from build123d import *

# Parameters (mm, degrees)
BOSS_EXTRUDE1_DEPTH                                  = 5
SKETCH2_W                                            = 20
SKETCH2_H                                            = 6
BOSS_EXTRUDE2_DEPTH                                  = 30
SKETCH3_R                                            = 1.5
CUT_EXTRUDE1_DEPTH                                   = 50.558046773
REFRENTADO_PARA_TORNILLO_CON_CABEZA_PLAN_D           = 3.4
REFRENTADO_PARA_TORNILLO_CON_CABEZA_PLAN_CBORE_D     = 6.5
REFRENTADO_PARA_TORNILLO_CON_CABEZA_PLAN_CBORE_DEPTH = 2
CUT_EXTRUDE2_REACH                                   = 47
SKETCH7_R                                            = 2.5
TALADRO_DE_MARGEN_PARA_M51_D                         = 5.3
TALADRO_DE_MARGEN_PARA_M51_DEPTH                     = 5
TALADRO_DE_MARGEN_PARA_M51_TIP                       = 1.59228064


with BuildPart() as part:
    # Sketch1 → Boss-Extrude1 (new body)
    with BuildSketch(Plane(origin=(0, 0, 0), x_dir=(1, 0, 0), z_dir=(0, 1, 0))):
        Polygon((0, 0), (-20, 0), (-20, -20), (0, -20), (20, -20), (20, 0), (20, 20), (0, 20), align=None)
    extrude(amount=-BOSS_EXTRUDE1_DEPTH)

    # Sketch2 → Boss-Extrude2 (add)
    with BuildSketch(Plane(origin=(0, 0, 0), x_dir=(1, 0, 0), z_dir=(0, 1, 0))):
        with Locations((10, 17)):
            Rectangle(SKETCH2_W, SKETCH2_H)
    extrude(amount=BOSS_EXTRUDE2_DEPTH)

    # Sketch3 → Cut-Extrude1 (cut, through all)
    with BuildSketch(Plane.XY.offset(-14)):
        with Locations((2.5, 7)):
            Circle(SKETCH3_R)
        with Locations(Location((2.5, 23, 0), (0, 0, 180))):
            Circle(SKETCH3_R)
        with Locations(Location((17.5, 7, 0), (0, 0, 180))):
            Circle(SKETCH3_R)
        with Locations((17.5, 23)):
            Circle(SKETCH3_R)
    extrude(amount=-CUT_EXTRUDE1_DEPTH, mode=Mode.SUBTRACT)

    # Refrentado para tornillo con cabeza plana de M31 (through all)
    with Locations(Plane.XY.offset(-14)):
        with Locations((2.5, 23), (2.5, 7), (17.5, 7), (17.5, 23)):
            CounterBoreHole(REFRENTADO_PARA_TORNILLO_CON_CABEZA_PLAN_D / 2, REFRENTADO_PARA_TORNILLO_CON_CABEZA_PLAN_CBORE_D / 2, REFRENTADO_PARA_TORNILLO_CON_CABEZA_PLAN_CBORE_DEPTH)

    # Sketch7 → Cut-Extrude2 (cut, up to next)
    with BuildSketch(Plane.XZ.offset(5), mode=Mode.PRIVATE) as cut_extrude2_sk1:
        with Locations(Location((-10, 10, 0), (0, 0, 270))):
            Circle(SKETCH7_R)
    cut_extrude2_tool1 = extrude(cut_extrude2_sk1.sketch, amount=-CUT_EXTRUDE2_REACH, mode=Mode.PRIVATE) & part.part
    add(cut_extrude2_tool1.solids().sort_by_distance((-10, -5, 10))[0], mode=Mode.SUBTRACT)

    # Taladro de margen para M51
    with Locations(Plane(origin=(0, -5, 0), x_dir=(-1, 0, 0), z_dir=(0, -1, 0))):
        with Locations((10, -10)):
            Hole(TALADRO_DE_MARGEN_PARA_M51_D / 2, depth=TALADRO_DE_MARGEN_PARA_M51_DEPTH)
            with Locations((0, 0, -(TALADRO_DE_MARGEN_PARA_M51_DEPTH + TALADRO_DE_MARGEN_PARA_M51_TIP / 2))):  # 118° drill point
                Cone(0, TALADRO_DE_MARGEN_PARA_M51_D / 2, TALADRO_DE_MARGEN_PARA_M51_TIP, mode=Mode.SUBTRACT)


solid = part.part
Model file for the job. Use its own axes, mm. A direction names the side the tool comes from. Give positions to 0.01 mm unless a question says otherwise; leave off trailing zeros. Write each loop counter-clockwise with the first axis right and the second up, starting at its lowest first coordinate (ties: lowest second). Pieces come first, ordered by that corner, then holes. Notation, with made-up numbers: M 82,16.25 L 116,16.25 A13 cw 116,27.25 Z; hole C -12.5,65 d9. An arc over 180 degrees is marked long. One line per item, written item: value. Start each with the question number.
Q1. Probe probe 1 along Y at (x, z) = (2.5, -14.85); probe 2 along X at (y, z) = (-1, -3); probe 3 along Z at (x, y) = (2, 17.5). List the from-to ranges inside material, lowest first. Write a range as [from, to].
Q2. Saw through at C-C, the plane x = 2.5. Write the cut outline in (y, z).
Q3. Saw through at D-D, the plane z = -18. Write the cut outline in (x, y), plus the area to 3 significant figures.
Q4. Saw through at A-A, the plane x = -10. Write the cut outline in (y, z), plus the area to 3 significant figures.
Q5. Drop flat-ended pins along their axis: pin 1 Ø2.5 at (x, y) = (-13, -3) entering from -Z; pin 2 Ø10.5 at (x, y) = (2.5, 7) entering from +Z; pin 3 Ø3 at (x, y) = (18, 5.5) entering from +Z. Give the stop position or say it passes through.
Q6. Two-plate mould, pull along X, no slides. Class faces 1 (the cylindrical face through (14.25, 23.11, -14.99)), 2 (the flat face through (4, 0, 7)), 3 (the flat face through (-20, -2, 10)): +X half, -X half, draft (parallel to the pull), parting line (faces both ways), or undercut.
Q7. Saw through at B-B, the plane y = 23. Write the cut outline in (x, z), plus the area to 3 significant figures.
Q8. 3-axis set-ups, long thin cutter, end or side, ignore diameter. For faces 4 (the flat face through (0, 8, -17)), 5 (the flat face through (0, -2, 20)), 6 (the flat face through (10, 15, -14)), 7 (the flat face through (10, 30, -17)), 8 (the flat face through (4.1, 21.6, -16)): which of +Z, -Z, +X, -X, +Y, -Y reach the whole face in a straight line?
Output values:
1. probe 1: y = [-5, 3.75], [10.25, 19.75], [26.25, 30]
1. probe 2: x = [0, 20]
1. probe 3: z = [-20, -14]
2. outline: M -5,-20 L 5.3,-20 L 5.3,-16 L 3.75,-16 L 3.75,-14 L 0,-14 L 0,20 L -5,20 Z; M 8.7,-20 L 21.3,-20 L 21.3,-16 L 19.75,-16 L 19.75,-14 L 10.25,-14 L 10.25,-16 L 8.7,-16 Z; M 24.7,-20 L 30,-20 L 30,-14 L 26.25,-14 L 26.25,-16 L 24.7,-16 Z
3. outline: M 0,-5 L 20,-5 L 20,30 L 0,30 Z; hole C 2.5,7 d3.4; hole C 2.5,23 d3.4; hole C 17.5,7 d3.4; hole C 17.5,23 d3.4
3. area: 664 mm²
4. outline: M -5,0 L 0,0 L 0,7.35 L -5,7.35 Z; M -5,12.65 L 0,12.65 L 0,20 L -5,20 Z
4. area: 73.5 mm²
5. pin 1: stops at z = 0
5. pin 2: stops at z = -14
5. pin 3: stops at z = -16
6. face 1: undercut
6. face 2: draft
6. face 3: -X half
7. outline: M 0,-20 L 0.8,-20 L 0.8,-16 L 0,-16 Z; M 4.2,-20 L 15.8,-20 L 15.8,-16 L 14.25,-16 L 14.25,-14 L 5.75,-14 L 5.75,-16 L 4.2,-16 Z; M 19.2,-20 L 20,-20 L 20,-16 L 19.2,-16 Z
7. area: 69.8 mm²
8. face 4: -Z, -X, +Y, -Y
8. face 5: +Z, +X, -X, +Y, -Y
8. face 6: +Z, +X, -X, +Y
8. face 7: +Z, -Z, +X, -X, +Y
8. face 8: +Z
